Geometry check sheet. Reference: the model listing, model coordinates, mm. A direction names the side the tool comes from. Coordinates: 2 decimals unless noted, no trailing zeros. Order: outer loops, then holes, each group sorted by start corner. A loop starts at its lowest first (then second) coordinate and runs counter-clockwise, first axis right, second up. Notation, with made-up numbers: (39.5, 8) - (76.5, 8) arc R10 ccw to (76.5, 18) - close; hole circle Ø11 at (23.25, -26). An arc over 180 degrees is marked (long way). One line per item, written item: value. Start each with the question number.
Autodesk Inventor part; units mm, degrees
ref_plane "YZ Plane" through (0, 0, 0) normal (1, 0, 0) x (0, 1, 0)
ref_plane "XZ Plane" through (0, 0, 0) normal (0, 1, 0) x (-1, 0, 0)
ref_plane "XY Plane" through (0, 0, 0) normal (0, 0, 1) x (1, 0, 0)
sketch "Boceto1" plane through (0, 0, 0) normal (0, 1, 0) x (-1, 0, 0)
  line L0 (100, 80) -> (-100, 80)
  line L1 (-100, 80) -> (-100, -80)
  line L2 (-100, -80) -> (100, -80)
  line L3 (100, -80) -> (100, 80)
  line L4 (100, 80) -> (-100, -80) construction
  line L5 (-100, 80) -> (100, -80) construction
  point P0 (0, 0)
  dimension "d0" = 200
  dimension "d1" = 160
extrude "Extrusión1" add sketch "Boceto1" along normal blind 20
sketch "Boceto2" plane through (0, 20, 0) normal (0, 1, 0) x (1, 0, 0)
  line L0 (-100, 80) -> (-100, -80)
  line L1 (-100, 80) -> (-70, 80)
  line L2 (-70, 80) -> (-70, 40)
  line L3 (-70, 40) -> (-100, 40)
  line L4 (-100, 40) -> (-100, 80)
  line L5 (100, 80) -> (-100, 80)
  line L6 (0, 80) -> (0, 40)
  line L7 (100, 80) -> (70, 80)
  line L8 (70, 80) -> (70, 40)
  line L9 (70, 40) -> (100, 40)
  line L10 (100, 40) -> (100, 80)
  point P0 (0, 0)
  dimension "d4" = 30
  dimension "d5" = 40
extrude "Extrusión2" cut sketch "Boceto2" against normal blind 10
sketch "Boceto3" plane through (0, 20, 0) normal (0, 1, 0) x (1, 0, 0)
  line L0 (-70, 80) -> (-70, 40)
  line L1 (-70, 80.0001) -> (-70, 40)
  line L2 (-70, 40) -> (-100, 40)
  line L3 (-100, 40) -> (-100, 80.0001)
  line L4 (-100, 40) -> (-70, 40)
  line L5 (-70, 40) -> (-70, 80)
  line L6 (-70, 80) -> (-100, 80)
  line L7 (-100, 80) -> (-100, 40)
  circle A0 centre (-88.25, 58.25) radius 1.75
  circle A1 centre (-81.75, 51.75) radius 1.75
  line L8 (100, 80) -> (-100, 80)
  line L9 (0, 80) -> (0, 56.5)
  circle A2 centre (88.25, 58.25) radius 1.75
  circle A3 centre (81.75, 51.75) radius 1.75
  point P0 (0, 0)
  point P1 (-64.3507, 80)
  point P2 (-74.3507, 0)
  point P3 (-85, 80)
  dimension "d23" = 21.75
  dimension "d24" = 11.75
  dimension "d26" = 11.75
hole "Agujero1" at (-81.75, 20, -51.75) at (-88.25, 20, -58.25) at (81.75, 20, -51.75) at (88.25, 20, -58.25) direction (0, -1, 0) diameter 3.5 end through all
sketch "Boceto4" plane through (-100, 0, 80) normal (0, 0, 1) x (1, 0, 0)
  line L0 (30, 20) -> (60, 20)
  line L1 (60, 20) -> (60, 10)
  line L2 (60, 10) -> (30, 10)
  line L3 (30, 10) -> (30, 20)
  line L4 (0, 0) -> (0, 20)
  line L5 (100, 0) -> (100, 10)
  line L6 (170, 20) -> (140, 20)
  line L7 (140, 20) -> (140, 10)
  line L8 (140, 10) -> (170, 10)
  line L9 (170, 10) -> (170, 20)
  dimension "d34" = 30
  dimension "d35" = 10
  dimension "d36" = 30
extrude "Extrusión3" add sketch "Boceto4" along normal blind 40
sketch "Boceto5" plane through (0, 20, 0) normal (0, 1, 0) x (1, 0, 0)
  line L0 (59.9999, -50) -> (69.9999, -50)
  line L1 (49.9999, -101.75) -> (49.9999, -79.9497)
  line L2 (59.9999, -108.25) -> (59.9999, -50)
  line L3 (40, -80) -> (69.9999, -80)
  line L4 (49.9999, -79.9497) -> (40, -80)
  circle A0 centre (51.7499, -101.75) radius 1.75
  circle A1 centre (58.2499, -108.25) radius 1.75
  line L5 (69.9999, -80) -> (69.9999, -120)
  line L6 (40, -120) -> (40, -80)
  line L7 (69.9999, -120) -> (40, -120)
  line L8 (0, -50) -> (0, -71.75)
  line L9 (-40, -120) -> (-40, -80)
  line L10 (-49.9999, -101.75) -> (-49.9999, -79.9497)
  circle A2 centre (-51.7499, -101.75) radius 1.75
  circle A3 centre (-58.2499, -108.25) radius 1.75
  line L11 (-40, -80) -> (-69.9999, -80)
  line L12 (-69.9999, -120) -> (-40, -120)
  line L13 (-69.9999, -80) -> (-69.9999, -120)
  line L14 (-59.9999, -108.25) -> (-59.9999, -50)
  line L15 (-40, -120) -> (-69.9999, -120)
  line L16 (-69.9999, -80) -> (-69.9999, -120)
  line L17 (-40, -120) -> (-70, -120)
  line L18 (-40, -80) -> (-40, -120)
  line L19 (-59.9999, -110) -> (-49.9999, -110)
  line L20 (-49.9999, -110) -> (-49.9999, -100)
  line L21 (-49.9999, -100) -> (-59.9999, -100)
  line L22 (-59.9999, -100) -> (-59.9999, -110)
  line L23 (-100, 40) -> (-100, -80)
  point P0 (0, 0)
  point P1 (-56.75, -68.25)
  point P2 (-63.25, -61.75)
  point P3 (63.25, -61.75)
  point P4 (56.75, -68.25)
  dimension "d45" = 3.5
  dimension "d46" = 3.5
  dimension "d39" = 10
  dimension "d40" = 10
  dimension "d41" = 40
  dimension "d42" = 0
  dimension "d43" = 6.5
  dimension "d44" = 6.5
  dimension "d47" = 11.7499
  dimension "d48" = 11.75
  dimension "d49" = 0
  dimension "d50" = 11.75
  dimension "d51" = 0
  dimension "d97" = 40.0001
hole "Agujero2" at (-58.2499, 20, 108.25) at (-51.7499, 20, 101.75) at (51.7499, 20, 101.75) at (58.2499, 20, 108.25) direction (0, -1, 0) diameter 3.5 end through all
sketch "Boceto6" plane through (0, 20, 0) normal (0, 1, 0) x (1, 0, 0)
  circle A0 centre (-60.569, -13.1067) radius 10
  circle A1 centre (-29.569, -59.1067) radius 3.5
  line L0 (-60.569, -13.1067) -> (-39.0083, -13.1067)
  circle A2 centre (-29.569, 25.8933) radius 3.5
  circle A3 centre (-88.569, 25.8933) radius 3.5
  circle A4 centre (-88.569, -59.1067) radius 3.5
  line L1 (8.592, 54.4846) -> (60.592, 54.4846)
  line L2 (60.592, 54.4846) -> (60.592, -15.5154)
  line L3 (60.592, -15.5154) -> (8.592, -15.5154)
  line L4 (8.592, -15.5154) -> (8.592, 54.4846)
  line L5 (8.592, -15.5154) -> (30.592, -15.5154)
  line L6 (30.592, -15.5154) -> (30.592, -57.5154)
  line L7 (30.592, -57.5154) -> (8.592, -57.5154)
  line L8 (8.592, -57.5154) -> (8.592, -15.5154)
  line L9 (1.8175, -0.4091) -> (1.8182, -2.9066)
  circle A5 centre (15.2757, -2.8065) radius 1.75
  line L10 (8.2823, 15.5794) -> (8.2823, -30.8467)
  circle A6 centre (43.2156, -2.8061) radius 1.75
  line L11 (53.8882, 4.6711) -> (53.8882, 2.1733)
  circle A7 centre (10.1956, 49.2639) radius 1.75
  line L12 (52.6186, -43.5722) -> (52.6186, -46.0699)
  circle A8 centre (58.4389, 47.9943) radius 1.75
  line L13 (60.3523, 47.3505) -> (8.2823, 47.3505)
  line L14 (60.3523, 47.3505) -> (60.3523, -0.8928)
  line L15 (34.3173, 47.3505) -> (34.3173, 23.2289)
  point P0 (0, 0)
  point P1 (-60.569, -16.6067)
  point P2 (33.6213, -21.4557)
  dimension "d59" = 7
  dimension "d60" = 7
  dimension "d61" = 7
  dimension "d62" = 39
  dimension "d63" = 46
  dimension "d64" = 59
  dimension "d65" = 46
  dimension "d66" = 39
  dimension "d67" = 59
  dimension "d68" = 52
  dimension "d69" = 70
  dimension "d70" = 22
  dimension "d71" = 42
  dimension "d72" = 3.5
  dimension "d73" = 3.5
  dimension "d74" = 3.5
  dimension "d75" = 3.5
hole "Agujero3" at (10.1956, 20, -49.2639) at (58.4389, 20, -47.9943) at (15.2757, 20, 2.8065) at (43.2156, 20, 2.8061) direction (0, -1, 0) diameter 3.5 end through all
sketch "Boceto7" plane through (0, 20, 0) normal (0, 1, 0) x (1, 0, 0)
  circle A0 centre (-60.569, -13.1067) radius 10
  circle A1 centre (-29.569, -59.1067) radius 3.5
  line L0 (-60.569, -13.1067) -> (-39.0083, -13.1067)
  circle A2 centre (-29.569, 25.8933) radius 3.5
  circle A3 centre (-88.569, 25.8933) radius 3.5
  circle A4 centre (-88.569, -59.1067) radius 3.5
  point P0 (0, 0)
  point P1 (-60.569, -16.6067)
  dimension "d83" = 7
  dimension "d84" = 7
  dimension "d85" = 7
  dimension "d86" = 39
  dimension "d87" = 46
  dimension "d88" = 59
  dimension "d89" = 46
  dimension "d90" = 39
  dimension "d91" = 59
extrude "Extrusión4" cut sketch "Boceto7" against normal blind 20
properties part number "base_mid_20"
Q1. Gauge pin test, flat ends, axial feed: P1, Ø3, axis at x = 58.25, z = 108.25, coming from the -Y side; P2, Ø6, axis at x = -79, y = 9.5, coming from the +Z side; P3, Ø9, axis at x = -85.5, z = -65.5, coming from the +Y side; P4, Ø3, axis at x = -88, y = 14, coming from the -Z side. Record the tip position at first contact, or that the pin passes through.
Q2. Cross-section at B-B, the plane x = 23. Enter the section's corners in (y, z), and give its area (3 significant figures).
Q3. Cross-section at A-A, the plane y = 14.75. Count the separate pieces of the cut face and the enclosed holes in it, and give its area (3 significant figures).
Q4. Material ranges on probe 1 along Z at (x, y) = (-88.25, 3.75); probe 2 along X at (y, z) = (16.5, 101.75); probe 3 along Z at (x, y) = (28, 9.25), recorded low to high.
Q5. Release check for a two-part mould opening along Z. For faces 4 (the flat face through (85, 15, -40)), 5 (the flat face through (70, 15, 100)), 6 (the cylindrical face through (-91.346, 10.14, 61.236)) record: released by +Z, released by -Z, zero draft, split by the parting line, or undercut.
Q6. Set-up check for faces 1 (the flat face through (40, 15, 100)), 2 (the flat face through (-55, 10, 100)), 3 (the flat face through (-70, 15, 100)): record each of +Z, -Z, +X, -X, +Y, -Y from which the full face is reachable in a straight line by a thin tool's end or side.
Check result:
1. P1: passes through
1. P2: stops at z = 80
1. P3: stops at y = 10
1. P4: stops at z = -40
2. outline: (0, -80) - (20, -80) - (20, 80) - (0, 80) - close
2. area: 3,200 mm2
3. separate pieces: 1
3. enclosed holes: 13
3. area: 31,500 mm2
4. probe 1: z = -80 to -60, -56.5 to -29.38, -22.41 to 55.62, 62.59 to 80
4. probe 2: x = -70 to -53.5, -50 to -40, 40 to 50, 53.5 to 70
4. probe 3: z = -80 to 80
5. face 4: released by -Z
5. face 5: zero draft
5. face 6: undercut
6. face 1: +Z, +Y, -Y
6. face 2: +Z, +X, -X, -Y
6. face 3: +Z, -X, +Y, -Y
